from build123d import *

# Parameters (mm, degrees)
SKETCH1_R                        = 2.15
MAIN_DEPTH                       = 4
WIRE_ESCAPES_REACH               = 120.496
SKETCH4_W                        = 7
SKETCH4_H                        = 30
BUTTON_CLEARANCE_REACH           = 120.496
SKETCH5_W                        = 80
SKETCH5_H                        = 10.8
M2_HEAT_SETS_D                   = 2.9
M2_HEAT_SETS_CBORE_D             = 3.3
M2_HEAT_SETS_CBORE_DEPTH         = 0.3
SKETCH7_W                        = 10
SKETCH7_H                        = 10
ENCODER_STANDOFF_DEPTH           = 1
SKETCH9_W                        = 8.7
SKETCH9_H                        = 5.7
ENCODER_TERMINAL_CLEARANCE_DEPTH = 2
FILLET1_R                        = 1


with BuildPart() as part:
    # Sketch1 → Main (new body)
    with BuildSketch(Plane(origin=(0, 0, 0), x_dir=(1, 0, 0), z_dir=(0, 1, 0))):
        Polygon((0, 0), (-102.8, 0), (-102.8, -53.8), (-97.4, -53.8), (-97.4, -58.8), (-15.4, -58.8), (-15.4, -53.8), (0, -53.8), align=None)
        with Locations(Location((-97.9, -4.9, 0), (0, 0, 270))):
            Circle(SKETCH1_R, mode=Mode.SUBTRACT)
        with Locations(Location((-97.9, -48.9, 0), (0, 0, 270))):
            Circle(SKETCH1_R, mode=Mode.SUBTRACT)
        with Locations(Location((-4.9, -4.9, 0), (0, 0, 270))):
            Circle(SKETCH1_R, mode=Mode.SUBTRACT)
        with Locations(Location((-4.9, -48.9, 0), (0, 0, 270))):
            Circle(SKETCH1_R, mode=Mode.SUBTRACT)
    extrude(amount=MAIN_DEPTH)

    # Sketch4 → Wire Escapes (cut, up to next)
    with BuildSketch(Plane(origin=(0, 4, 0), x_dir=(1, 0, 0), z_dir=(0, 1, 0)), mode=Mode.PRIVATE) as wire_escapes_sk1:
        with Locations((-99.3, -28.8)):
            Rectangle(SKETCH4_W, SKETCH4_H)
    wire_escapes_tool1 = extrude(wire_escapes_sk1.sketch, amount=-WIRE_ESCAPES_REACH, mode=Mode.PRIVATE) & part.part
    add(wire_escapes_tool1.solids().sort_by_distance((-99.3, 4, 28.8))[0], mode=Mode.SUBTRACT)

    # Sketch5 → Button Clearance (cut, up to next)
    with BuildSketch(Plane(origin=(0, 4, 0), x_dir=(1, 0, 0), z_dir=(0, 1, 0)), mode=Mode.PRIVATE) as button_clearance_sk1:
        with Locations((-51.4, -5.4)):
            Rectangle(SKETCH5_W, SKETCH5_H)
    button_clearance_tool1 = extrude(button_clearance_sk1.sketch, amount=-BUTTON_CLEARANCE_REACH, mode=Mode.PRIVATE) & part.part
    add(button_clearance_tool1.solids().sort_by_distance((-51.4, 4, 5.4))[0], mode=Mode.SUBTRACT)

    # M2 Heat Sets (through all)
    with Locations(Plane(origin=(-90.8, 4, 16.05), x_dir=(0, 0, 1), z_dir=(0, 1, 0))):
        with Locations((0, 0), (38.04, 0), (38.04, 65.46), (0, 65.46), (4.95, 72.125), (19.35, 72.125)):
            CounterBoreHole(M2_HEAT_SETS_D / 2, M2_HEAT_SETS_CBORE_D / 2, M2_HEAT_SETS_CBORE_DEPTH)

    # Sketch7 → Encoder Standoff (add)
    with BuildSketch(Plane(origin=(0, 4, 0), x_dir=(1, 0, 0), z_dir=(0, 1, 0))):
        with Locations((-9.8375, -26.5)):
            Rectangle(SKETCH7_W, SKETCH7_H)
    extrude(amount=ENCODER_STANDOFF_DEPTH)

    # Sketch9 → Encoder Terminal Clearance (cut)
    with BuildSketch(Plane(origin=(0, 4, 0), x_dir=(1, 0, 0), z_dir=(0, 1, 0))):
        with Locations((-11.35, -18.65)):
            Rectangle(SKETCH9_W, SKETCH9_H)
        Polygon((-15.7, -31.5), (-7, -31.5), (-7, -38.4), (-3, -38.4), (-3, -42.4), (-18.5, -42.4), (-18.5, -38.4), (-15.7, -38.4), align=None)
    extrude(amount=-ENCODER_TERMINAL_CLEARANCE_DEPTH, mode=Mode.SUBTRACT)

    # Fillet1
    # the kernel refuses this fillet: 1 mm, written as the material it adds along each edge
    with BuildSketch(Plane(origin=(-15.4, 0, 53.8), x_dir=(1, 0, 0), z_dir=(0, 1, 0)), Plane(origin=(-97.4, 0, 53.8), x_dir=(0, 0, 1), z_dir=(0, 1, 0)), Plane(origin=(-11.4, 4, 10.8), x_dir=(0, 0, -1), z_dir=(0, -1, 0)), Plane(origin=(-91.4, 4, 10.8), x_dir=(1, 0, 0), z_dir=(0, -1, 0))) as fillet1_piece_1:
        with BuildLine():
            CenterArc((FILLET1_R, -FILLET1_R), FILLET1_R, 90, 90)
            Line((0, -FILLET1_R), (0, 0))
            Line((0, 0), (FILLET1_R, 0))
        make_face()
    extrude(amount=4)
    with BuildSketch(Plane(origin=(-95.8, 4, 43.8), x_dir=(-1, 0, 0), z_dir=(0, -1, 0)), Plane(origin=(-95.8, 4, 13.8), x_dir=(0, 0, 1), z_dir=(0, -1, 0))) as fillet1_piece_2:
        with BuildLine():
            CenterArc((FILLET1_R, FILLET1_R), FILLET1_R, 180, 90)
            Line((0, FILLET1_R), (0, 0))
            Line((0, 0), (FILLET1_R, 0))
        make_face()
    extrude(amount=4)
    with BuildSketch(Plane(origin=(-18.5, 4, 42.4), x_dir=(0, 0, -1), z_dir=(0, -1, 0)), Plane(origin=(-3, 4, 42.4), x_dir=(-1, 0, 0), z_dir=(0, -1, 0)), Plane(origin=(-3, 4, 38.4), x_dir=(0, 0, 1), z_dir=(0, -1, 0)), Plane(origin=(-18.5, 4, 38.4), x_dir=(1, 0, 0), z_dir=(0, -1, 0)), Plane(origin=(-7, 4, 15.8), x_dir=(0, 0, 1), z_dir=(0, -1, 0)), Plane(origin=(-15.7, 4, 15.8), x_dir=(1, 0, 0), z_dir=(0, -1, 0)), Plane(origin=(-15.7, 4, 31.5), x_dir=(1, 0, 0), z_dir=(0, -1, 0)), Plane(origin=(-7, 4, 21.5), x_dir=(-1, 0, 0), z_dir=(0, -1, 0))) as fillet1_piece_3:
        with BuildLine():
            CenterArc((FILLET1_R, FILLET1_R), FILLET1_R, 180, 90)
            Line((0, FILLET1_R), (0, 0))
            Line((0, 0), (FILLET1_R, 0))
        make_face()
    extrude(amount=2)
    with BuildSketch(Plane(origin=(-15.7, 6.5, 21.5), x_dir=(1, 0, 0), z_dir=(0, -1, 0))) as fillet1_piece_4_section:
        with BuildLine():
            CenterArc((FILLET1_R, -FILLET1_R), FILLET1_R, 90, 90)
            Line((0, -FILLET1_R), (0, 0))
            Line((0, 0), (FILLET1_R, 0))
        make_face()
    fillet1_piece_4 = extrude(amount=4.5, mode=Mode.PRIVATE)
    fillet1_piece_4 = split(fillet1_piece_4, bisect_by=Plane(origin=(-14.8375, 4.5, 21.497152865), z_dir=(1, 0, 0)), keep=Keep.TOP, mode=Mode.PRIVATE)
    fillet1_piece_4 = split(fillet1_piece_4, bisect_by=Plane(origin=(-14.803157734, 5, 21.497152865), z_dir=(0, -1, 0)), keep=Keep.TOP, mode=Mode.PRIVATE)
    add(fillet1_piece_4)
    with BuildSketch(Plane(origin=(-15.7, 4, 21.5), x_dir=(1, 0, 0), z_dir=(0, -1, 0)), Plane(origin=(-7, 4, 31.5), x_dir=(-1, 0, 0), z_dir=(0, -1, 0))) as fillet1_piece_5:
        with BuildLine():
            CenterArc((FILLET1_R, -FILLET1_R), FILLET1_R, 90, 90)
            Line((0, -FILLET1_R), (0, 0))
            Line((0, 0), (FILLET1_R, 0))
        make_face()
    extrude(amount=2)
    with BuildSketch(Plane(origin=(-15.7, 6.5, 31.5), x_dir=(1, 0, 0), z_dir=(0, -1, 0))) as fillet1_piece_6_section:
        with BuildLine():
            CenterArc((FILLET1_R, FILLET1_R), FILLET1_R, 180, 90)
            Line((0, FILLET1_R), (0, 0))
            Line((0, 0), (FILLET1_R, 0))
        make_face()
    fillet1_piece_6 = extrude(amount=4.5, mode=Mode.PRIVATE)
    fillet1_piece_6 = split(fillet1_piece_6, bisect_by=Plane(origin=(-14.8375, 4.5, 31.502847135), z_dir=(1, 0, 0)), keep=Keep.TOP, mode=Mode.PRIVATE)
    fillet1_piece_6 = split(fillet1_piece_6, bisect_by=Plane(origin=(-14.803157734, 5, 31.502847135), z_dir=(0, -1, 0)), keep=Keep.TOP, mode=Mode.PRIVATE)
    add(fillet1_piece_6)
    # the kernel refuses this fillet: 1 mm, written as the material it takes off along each edge
    with BuildSketch(Plane(origin=(0, -2.5, 0), x_dir=(-1, 0, 0), z_dir=(0, 1, 0)), Plane(origin=(0, -2.5, 53.8), x_dir=(0, 0, -1), z_dir=(0, 1, 0)), Plane(origin=(-102.8, -2.5, 0), x_dir=(0, 0, 1), z_dir=(0, 1, 0)), Plane(origin=(-15.4, -2.5, 58.8), x_dir=(0, 0, -1), z_dir=(0, 1, 0)), Plane(origin=(-102.8, -2.5, 53.8), x_dir=(1, 0, 0), z_dir=(0, 1, 0)), Plane(origin=(-97.4, -2.5, 58.8), x_dir=(1, 0, 0), z_dir=(0, 1, 0)), Plane(origin=(-11.4, 6.5, 0), x_dir=(1, 0, 0), z_dir=(0, -1, 0))) as fillet1_2_piece_1:
        with BuildLine():
            CenterArc((FILLET1_R, FILLET1_R), FILLET1_R, 180, 90)
            Line((0, FILLET1_R), (0, 0))
            Line((0, 0), (FILLET1_R, 0))
        make_face()
    extrude(amount=9, mode=Mode.SUBTRACT)
    with BuildSketch(Plane(origin=(-102.8, 6.5, 43.8), x_dir=(0, 0, 1), z_dir=(0, -1, 0)), Plane(origin=(-102.8, 6.5, 13.8), x_dir=(1, 0, 0), z_dir=(0, -1, 0)), Plane(origin=(-91.4, 6.5, 0), x_dir=(-1, 0, 0), z_dir=(0, -1, 0))) as fillet1_2_piece_2:
        with BuildLine():
            CenterArc((FILLET1_R, -FILLET1_R), FILLET1_R, 90, 90)
            Line((0, -FILLET1_R), (0, 0))
            Line((0, 0), (FILLET1_R, 0))
        make_face()
    extrude(amount=9, mode=Mode.SUBTRACT)
    with BuildSketch(Plane(origin=(-4.8375, 4, 21.5), x_dir=(0, 0, 1), z_dir=(0, 1, 0)), Plane(origin=(-4.8375, 4, 31.5), x_dir=(-1, 0, 0), z_dir=(0, 1, 0))) as fillet1_2_piece_3:
        with BuildLine():
            CenterArc((FILLET1_R, -FILLET1_R), FILLET1_R, 90, 90)
            Line((0, -FILLET1_R), (0, 0))
            Line((0, 0), (FILLET1_R, 0))
        make_face()
    extrude(amount=3.5, mode=Mode.SUBTRACT)
    with BuildSketch(Plane(origin=(-15.7, 6.5, 38.4), x_dir=(-1, 0, 0), z_dir=(0, -1, 0))) as fillet1_2_piece_4:
        with BuildLine():
            CenterArc((FILLET1_R, FILLET1_R), FILLET1_R, 180, 90)
            Line((0, FILLET1_R), (0, 0))
            Line((0, 0), (FILLET1_R, 0))
        make_face()
    extrude(amount=4.5, mode=Mode.SUBTRACT)
    with BuildSketch(Plane(origin=(-7, 6.5, 38.4), x_dir=(1, 0, 0), z_dir=(0, -1, 0))) as fillet1_2_piece_5:
        with BuildLine():
            CenterArc((FILLET1_R, -FILLET1_R), FILLET1_R, 90, 90)
            Line((0, -FILLET1_R), (0, 0))
            Line((0, 0), (FILLET1_R, 0))
        make_face()
    extrude(amount=4.5, mode=Mode.SUBTRACT)


solid = part.part
The listing builds one solid part. Answer for the finished solid, in the listing's coordinates (mm). A direction names the side the tool comes from. Give positions to 0.01 mm unless a question says otherwise; leave off trailing zeros. Write each loop counter-clockwise with the first axis right and the second up, starting at its lowest first coordinate (ties: lowest second). Pieces come first, ordered by that corner, then holes.
Item 1: Determine the mould class of faces 1 (the flat face through (-10, 5, 27)), 2 (the flat face through (-7, 3, 19)), 3 (the flat face through (-6, 2, 0)), 4 (the flat face through (-18.5, 3, 40)) for opening direction Z: released by +Z, released by -Z, zero draft, split by the parting line, or undercut.
Item 2: Which of the six approach directions +Z, -Z, +X, -X, +Y, -Y give full straight-line access (tool end or side, diameter ignored) to faces 5 (the flat face through (-11.4, 2, 5)), 6 (the flat face through (-15.4, 2, 56)), 7 (the flat face through (-100, 2, 53.8))?
Item 3: Section C-C, the plane z = 4.9 is taken. Write down the section's boundary in (x, y).
Item 4: Section D-D, the plane z = 35.4 is taken. Write down the section's boundary in (x, y) (3 decimals), plus the area to 3 significant figures.
Item 5: Flat-ended cylindrical pins translate along their axes: P1, Ø4.5, axis at x = -90.8, z = 16.05, coming from the -Y side; P2, Ø1.5, axis at x = -67.5, y = 1, coming from the -Z side; P3, Ø1.5, axis at y = 1.5, z = 56.5, coming from the -X side; P4, Ø1.2, axis at x = -7, y = 2, coming from the +Z side. Find the tip coordinate at first contact, or state that the pin passes through.
Item 6: Section A-A, the plane x = -25.34 is taken. Write down the section's boundary in (y, z), plus the area to 3 significant figures.
Item 7: Find the intervals of material crossed by line 1 along X through (y, z) = (1.2, 16.05); line 2 along X through (y, z) = (1.8, 56.5); line 3 along Y through (x, z) = (-15.5, 15), in increasing order.
Item 8: Section B-B, the plane z = 50 is taken. Write down the section's boundary in (x, y), plus the area to 3 significant figures.
Completed:
1. face 1: zero draft
1. face 2: undercut
1. face 3: released by -Z
1. face 4: undercut
2. face 5: -Z, +Y, -Y
2. face 6: +Z, +X, +Y, -Y
2. face 7: +Z, -X, +Y, -Y
3. outline: (-102.8, 0) - (-100.05, 0) - (-100.05, 4) - (-102.8, 4) - close; (-95.75, 0) - (-91.4, 0) - (-91.4, 4) - (-95.75, 4) - close; (-11.4, 0) - (-7.05, 0) - (-7.05, 4) - (-11.4, 4) - close; (-2.75, 0) - (0, 0) - (0, 4) - (-2.75, 4) - close
4. outline: (-95.8, 0) - (-20.125, 0) - (-20.125, 3.7) - (-20.325, 3.7) - (-20.325, 4) - (-95.8, 4) - close; (-17.225, 0) - (0, 0) - (0, 4) - (-7, 4) - (-7, 2) - (-15.7, 2) - (-15.7, 4) - (-17.025, 4) - (-17.025, 3.7) - (-17.225, 3.7) - close
4. area: 354 mm2
5. P1: stops at y = 0
5. P2: stops at z = 10.8
5. P3: stops at x = -97.4
5. P4: stops at z = 53.8
6. outline: (0, 10.8) - (4, 10.8) - (4, 14.4) - (3.7, 14.4) - (3.7, 14.6) - (0, 14.6) - close; (0, 17.5) - (3.7, 17.5) - (3.7, 17.7) - (4, 17.7) - (4, 52.44) - (3.7, 52.44) - (3.7, 52.64) - (0, 52.64) - close; (0, 55.54) - (3.7, 55.54) - (3.7, 55.74) - (4, 55.74) - (4, 58.8) - (0, 58.8) - close
6. area: 169 mm2
7. line 1: x = -95.8 to -92.25, -89.35 to -26.79, -23.89 to 0
7. line 2: x = -97.4 to -15.4
7. line 3: y = 0 to 4
8. outline: (-102.8, 0) - (-99.75, 0) - (-99.75, 4) - (-102.8, 4) - close; (-96.05, 0) - (-6.75, 0) - (-6.75, 4) - (-96.05, 4) - close; (-3.05, 0) - (0, 0) - (0, 4) - (-3.05, 4) - close
8. area: 382 mm2
